The listing builds one solid part. Answer for the finished solid, in the listing's coordinates (mm). A direction names the side the tool comes from. Give positions to 0.01 mm unless a question says otherwise; leave off trailing zeros. Loops run counter-clockwise (first coordinate to the right, second up) from the corner with the lowest first, then second, coordinate; pieces in that order, holes last. Notation, with made-up numbers: M 52,-1 L 64,-1 A16 cw 64,17 Z; hole C 80,59.25 d11. An arc over 180 degrees is marked long. Return JSON: item names as keys, results as strings.
from build123d import *

# Parameters (mm, degrees)
F3_R     = 18.8713
F4_DEPTH = 41.148


with BuildPart() as f2:
    # F0 (on Front) → F2 (revolve)
    with BuildSketch(Plane.XZ):
        Polygon((-32.833509, 14.089718), (-51.704809, 41.12158), (-51.704809, 14.089718), align=None)
    revolve(axis=Axis((-51.704809, 0, 27.223122), (0, 0, -1)))

    # F3 (on face) → F4 (join)
    with BuildSketch(Plane(origin=(0, 0, 14.089718), x_dir=(1, 0, 0), z_dir=(0, 0, -1))):
        with Locations((-51.704809, 0)):
            Circle(F3_R)
    extrude(amount=F4_DEPTH)

    # F5 (on Front) → F6 (revolve)
    with BuildSketch(Plane.XZ):
        Polygon((-67.939401, -21.689953), (-67.712404, 7.753583), (-86.05796, -21.689953), align=None)
    revolve(axis=Axis((-51.704809, 0, 12.922877), (0, 0, 1)))


solid = f2.part
(1) Given pin 1 (12 mm diameter, centred on x = -69.5, y = -23.5, fed in from -Z); pin 2 (8 mm diameter, centred on x = -51.5, y = -23.5, fed in from +Z); pin 3 (10 mm diameter, centred on x = -62.5, z = 25, fed in from +Y), each flat-ended and moving along its own axis, determine where each tip first touches the part or whether it passes through.
Values follow:
{"pin 1": "z = -21.69", "pin 2": "z = 2.15", "pin 3": "y = 11.69"}
(2) Straight lines are drawn through the part: line 1 along X through (y, z) = (-24, -9); line 2 along Y through (x, z) = (-34.5, 9.5); line 3 along X through (y, z) = (-5, -18). For each, find the intervals that lie inside material, in ascending order.
Values follow:
{"line 1": "-62.81 to -40.6", "line 2": "-7.75 to 7.75", "line 3": "-83.37 to -20.04"}
(3) The part is cut by section A-A (z = 16.5). Determine the outline of the cut face in (x, y), and give its area (3 significant figures).
Values follow:
{"outline": "C -51.7,0 d34.38", "area": "928 mm²"}
(4) A tool of negligible diameter and unlimited length cuts with its end or side. For faces 1 (the cylindrical face through (-66.68, 11.483, 8.7)), 2 (the cylindrical face through (-66.68, 11.483, -24.337)), 3 (the flat face through (-52, 0, -27.058)), from which of +Z, -Z, +X, -X, +Y, -Y can it reach the whole face along a straight path? Write none if from no direction.
Values follow:
{"face 1": "+Z", "face 2": "-Z", "face 3": "-Z, +X, -X, +Y, -Y"}
